Source: CAD feature listing. Evaluate the final solid. Frame: model axes, mm. Face numbers are marked on the shaded views. A direction names the side the tool comes from. Round coordinates to 2 decimals unless told otherwise and drop trailing zeros. Order: outer loops, then holes, each group sorted by start corner. A loop starts at its lowest first (then second) coordinate and runs counter-clockwise, first axis right, second up. Notation, with made-up numbers: M -17,43.5 L 8,43.5 A16 ccw 8,70.5 Z; hole C 67.25,36 d10. An arc over 180 degrees is marked long. Answer as CSV lines item,"result". Start each with the question number.
Item 1: Pull-direction query (X, two-part tool) for the marked faces 6, 7 and 8; classes: +X half, -X half, draft (parallel to the pull), parting line (faces both ways), or undercut.
Item 2: Line query: line 1 (Z direction, x = 33, y = -21); line 2 (Z direction, x = 44.5, y = -11.5); line 3 (X direction, y = -7, z = 27). Output: solid intervals per line, ascending. Write a range as [from, to].
Item 3: First-contact query: P1, Ø17, axis at x = 8, y = -22.5, coming from the +Z side; P2, Ø21, axis at y = -17, z = 44, coming from the -X side; P3, Ø13, axis at x = 100, y = -24, coming from the +Z side. Flat tips, straight axial feed; report the tip coordinate or a pass-through.
Item 4: Section query A-A on y = -18. Return the cut outline in (x, z).
Item 5: Section query C-C on x = 32.5. Return the cut outline in (y, z).
Item 6: Section query B-B on x = 90. Return the cut outline in (y, z), plus the area to 3 significant figures.
Item 7: Set-up query: the marked faces 1, 2, 3, 4 and 5. Return all of +Z, -Z, +X, -X, +Y, -Y with unobstructed straight access to the full face (end or side cutting, diameter ignored); none if empty.
Item 8: Section query D-D on z = 26. Return the cut outline in (x, y), plus the area to 3 significant figures.
from build123d import *

# Parameters (mm, degrees)
F1_DEPTH  = 42
F3_DEPTH  = 112.001
F4_R      = 9.5
F5_DEPTH  = 112.001
F7_DEPTH  = 3
F9_DEPTH  = 22
F11_DEPTH = 25


with BuildPart() as f1:
    # F0 (on Front) → F1 (new body)
    with BuildSketch(Plane.XZ):
        Polygon((0, 16), (0, 0), (133, 0), (133, 16), (43, 16), (43, 66), (21, 66), (21, 16), align=None)
    extrude(amount=F1_DEPTH)

    # F2 (on face) → F3 (cut, through all)
    with BuildSketch(Plane(origin=(21, 0, 0), x_dir=(0, -1, 0), z_dir=(-1, 0, 0))):
        with BuildLine():
            Line((0, 66), (0, 45))
            ThreePointArc((0, 45), (6.1507575951, 59.8492424049), (21, 66))
            Line((21, 66), (0, 66))
        make_face()
        with BuildLine():
            Line((42, 66), (21, 66))
            ThreePointArc((21, 66), (35.8492424049, 59.8492424049), (42, 45))
            Line((42, 45), (42, 66))
        make_face()
    extrude(amount=-F3_DEPTH, mode=Mode.SUBTRACT)

    # F4 (on face) → F5 (cut, through all)
    with BuildSketch(Plane(origin=(21, 0, 0), x_dir=(0, -1, 0), z_dir=(-1, 0, 0))):
        with Locations((21, 45)):
            Circle(F4_R)
    extrude(amount=-F5_DEPTH, mode=Mode.SUBTRACT)

    # F6 (on face) → F7 (join)
    with BuildSketch(Plane.XY.offset(16)):
        with BuildLine():
            Line((108, -8), (64, -8))
            ThreePointArc((64, -8), (51, -21), (64, -34))
            Line((64, -34), (108, -34))
            ThreePointArc((108, -34), (121, -21), (108, -8))
        make_face()
    extrude(amount=F7_DEPTH)

    # F8 (on Front) → F9 (join)
    with BuildSketch(Plane.XZ):
        with BuildLine():
            ThreePointArc((25.2109261421, 60.5), (13.122975019, 31.3171044574), (9, 0))
            Line((9, 0), (130, 0))
            Line((130, 0), (25.2109261421, 60.5))
        make_face()
    extrude(amount=-F9_DEPTH)

    # F10 (on face) → F11 (cut)
    with BuildSketch(Plane.XY.offset(19)):
        with BuildLine():
            Line((108, -14.5), (64, -14.5))
            ThreePointArc((64, -14.5), (57.5, -21), (64, -27.5))
            Line((64, -27.5), (108, -27.5))
            ThreePointArc((108, -27.5), (114.5, -21), (108, -14.5))
        make_face()
    extrude(amount=-F11_DEPTH, mode=Mode.SUBTRACT)


solid = f1.part
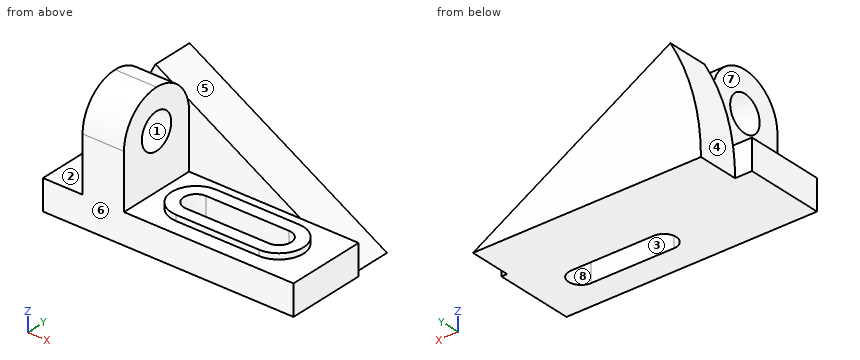
Results:
1,face 6,"draft"
1,face 7,"-X half"
1,face 8,"undercut"
2,line 1,"[0, 35.5], [54.5, 66]"
2,line 2,"[0, 16]"
2,line 3,"[21, 43]"
3,P1,"z = 16"
3,P2,"x = 21"
3,P3,"z = 19"
4,outline,"M 0,0 L 58.23,0 L 58.23,19 L 51.35,19 L 51.35,16 L 43,16 L 43,35.99 L 21,35.99 L 21,16 L 0,16 Z; M 21,54.01 L 43,54.01 L 43,65.78 L 21,65.78 Z; M 113.77,0 L 133,0 L 133,16 L 120.65,16 L 120.65,19 L 113.77,19 Z"
5,outline,"M -42,0 L 22,0 L 22,56.29 L 0,56.29 L 0,45 A21 ccw -42,45 Z; hole C -21,45 d19"
6,outline,"M -42,0 L -27.5,0 L -27.5,19 L -34,19 L -34,16 L -42,16 Z; M -14.5,0 L 22,0 L 22,23.09 L 0,23.09 L 0,16 L -8,16 L -8,19 L -14.5,19 Z"
6,area,"1,010 mm^2"
7,face 1,"+X, -X"
7,face 2,"+Z, -X, -Y"
7,face 3,"+Z, -Z"
7,face 4,"+Z, -X, +Y"
7,face 5,"+Z, +X, +Y"
8,outline,"M 11.83,0 L 21,0 L 21,-42 L 43,-42 L 43,0 L 84.97,0 L 84.97,22 L 11.83,22 Z"
8,area,"2,530 mm^2"
